Here's how the part is built. I have some questions about the finished solid (model axes, mm). A direction names the side the tool comes from. Coordinates: 2 decimals unless noted, no trailing zeros. Loops run counter-clockwise (first coordinate to the right, second up) from the corner with the lowest first, then second, coordinate; pieces in that order, holes last. Notation, with made-up numbers: (-31, 86.5) - (-26, 86.5) arc R35 ccw to (-26, 118.5) - close; hole circle Ø5 at (9, -16.5). An arc over 180 degrees is marked (long way). Use a Markdown table: item, result.
Autodesk Inventor part; units mm, degrees
ref_plane "YZ Plane" through (0, 0, 0) normal (1, 0, 0) x (0, 1, 0)
ref_plane "XZ Plane" through (0, 0, 0) normal (0, 1, 0) x (-1, 0, 0)
ref_plane "XY Plane" through (0, 0, 0) normal (0, 0, 1) x (1, 0, 0)
sketch "Sketch1" plane through (0, 0, 0) normal (0, 1, 0) x (-1, 0, 0)
  point P0 (0, 0)
sketch "Sketch2" plane through (0, 0, 0) normal (0, 1, 0) x (-1, 0, 0)
  line L0 (-76.2, 76.2) -> (76.2, 76.2)
  line L1 (76.2, 76.2) -> (76.2, -76.2)
  line L2 (76.2, -76.2) -> (-76.2, -76.2)
  line L3 (-76.2, -76.2) -> (-76.2, 76.2)
  line L4 (-76.2, 76.2) -> (76.2, -76.2) construction
  line L5 (76.2, 76.2) -> (-76.2, -76.2) construction
  point P0 (0, 0)
  dimension "d0" = 152.4
  dimension "d1" = 152.4
extrude "Extrusion1" add sketch "Sketch2" along normal blind 12.7
sketch "Sketch3" plane through (0, 12.7, 0) normal (0, 1, 0) x (1, 0, 0)
  line L0 (76.2, 76.2) -> (-76.2, 76.2)
  line L1 (76.2, -76.2) -> (76.2, 76.2)
  line L2 (-76.2, 76.2) -> (76.2, 76.2)
  line L3 (76.2, 76.2) -> (76.2, 63.5)
  line L4 (76.2, 63.5) -> (-76.2, 63.5)
  line L5 (-76.2, 63.5) -> (-76.2, 76.2)
  line L6 (-76.2, -76.2) -> (76.2, -76.2)
  line L7 (76.2, -76.2) -> (76.2, -63.5)
  line L8 (76.2, -63.5) -> (-76.2, -63.5)
  line L9 (-76.2, -63.5) -> (-76.2, -76.2)
  point P0 (0, 0)
  point P1 (76.2, -76.2)
  dimension "d4" = 12.7
  dimension "d5" = 12.7
  dimension "d15" = 152.4
extrude "Extrusion2" add sketch "Sketch3" along normal blind 127
fillet "Fillet1" radius 6.35 2 edges at (0, 0, 76.2) (0, 0, -76.2)
sketch "Sketch4" plane through (76.2, 12.7, -63.5) normal (1, 0, 0) x (0, 0, -1)
  circle A0 centre (-133.35, 120.65) radius 3.175
  circle A1 centre (-133.35, -6.35) radius 3.175
  circle A2 centre (-133.35, 57.15) radius 3.175
  circle A3 centre (6.35, 120.65) radius 3.175
  circle A4 centre (6.35, -6.35) radius 3.175
  circle A5 centre (6.35, 57.15) radius 3.175
  circle A6 centre (-63.5, -6.35) radius 3.175
  point P0 (-63.5, -12.7)
  dimension "d9" = 127
extrude "Extrusion3" cut sketch "Sketch4" against normal blind 12.7
sketch "Sketch5" plane through (-76.2, 12.7, 63.5) normal (-1, 0, 0) x (0, 0, 1)
  circle A0 centre (-133.35, 120.65) radius 3.175
  circle A1 centre (-133.35, 120.65) radius 3.175
  circle A2 centre (-133.35, 57.15) radius 3.175
  circle A3 centre (-133.35, 57.15) radius 3.175
  circle A4 centre (-133.35, -6.35) radius 3.175
  circle A5 centre (-133.35, -6.35) radius 3.175
  circle A6 centre (-63.5, -6.35) radius 3.175
  circle A7 centre (-63.5, -6.35) radius 3.175
  circle A8 centre (6.35, -6.35) radius 3.175
  circle A9 centre (6.35, -6.35) radius 3.175
  circle A10 centre (6.35, 57.15) radius 3.175
  circle A11 centre (6.35, 57.15) radius 3.175
  circle A12 centre (6.35, 120.65) radius 3.175
  circle A13 centre (6.35, 120.65) radius 3.175
  line L0 (6.35, -12.7) -> (-133.35, -12.7)
  point P0 (-63.5, -12.7)
  dimension "d20" = 69.85
sketch "Sketch6" plane through (0, 139.7, 0) normal (0, 1, 0) x (1, 0, 0)
  line L0 (76.2, 69.85) -> (-76.2, 69.85)
  circle A0 centre (0, 69.85) radius 3
  line L1 (-76.2, -69.85) -> (76.2, -69.85)
  circle A1 centre (0, -69.85) radius 3
  point P0 (0, 0)
  dimension "d16" = 6
  dimension "d17" = 6
extrude "Extrusion5" cut sketch "Sketch6" against normal blind 4
extrude "Extrusion6" cut sketch "Sketch5" against normal blind 12.7
properties part number "Fuselage_Body_Piece"
Q1. I want a section at A-A, the plane y = 133.35. Write out the boundary of the cut face in (x, z) (3 decimals).
Check values:
| item | result |
|---|---|
| outline | (-76.2, -76.2) - (76.2, -76.2) - (76.2, -73.025) - (63.5, -73.025) - (63.5, -66.675) - (76.2, -66.675) - (76.2, -63.5) - (-76.2, -63.5) - (-76.2, -66.675) - (-63.5, -66.675) - (-63.5, -73.025) - (-76.2, -73.025) - close; (-76.2, 63.5) - (76.2, 63.5) - (76.2, 66.675) - (63.5, 66.675) - (63.5, 73.025) - (76.2, 73.025) - (76.2, 76.2) - (-76.2, 76.2) - (-76.2, 73.025) - (-63.5, 73.025) - (-63.5, 66.675) - (-76.2, 66.675) - close |
Q2. I want a section at C-C, the plane z = 0. Write out the boundary of the cut face in (x, y) (3 decimals).
Check values:
| item | result |
|---|---|
| outline | (-76.2, 0) - (76.2, 0) - (76.2, 3.175) - (63.5, 3.175) - (63.5, 9.525) - (76.2, 9.525) - (76.2, 12.7) - (-76.2, 12.7) - (-76.2, 9.525) - (-63.5, 9.525) - (-63.5, 3.175) - (-76.2, 3.175) - close |
Q3. Which directions (+Z, -Z, +X, -X, +Y, -Y) give clear straight access to the entire face, cutting with the end or side of a thin tool? Please do faces 5 (the face through (63.5, 6, 70)), 6 (the face through (-69.94, 6.49, -73.02)), 7 (the face through (1, 75, 63.5)), 8 (the face through (0, 135.7, 70)).
Check values:
| item | result |
|---|---|
| face 5 | +X |
| face 6 | -X |
| face 7 | +X, -X, +Y |
| face 8 | +Y |
Q4. I want a section at B-B, the plane x = -9.5. Write out the boundary of the cut face in (y, z), then the cut area to 3 significant figures.
Check values:
| item | result |
|---|---|
| outline | (0, -69.85) arc R6.35 ccw to (6.35, -76.2) - (139.7, -76.2) - (139.7, -63.5) - (12.7, -63.5) - (12.7, 63.5) - (139.7, 63.5) - (139.7, 76.2) - (6.35, 76.2) arc R6.35 ccw to (0, 69.85) - close |
| area | 5,140 mm^2 |
Q5. Please list where these lines run through material, in increasing order: L1, parallel to Z at x = 73, y = 133; L2, parallel to Y at x = -67, z = -69.85 (3 decimals); L3, parallel to Z at x = 59.5, y = 43. Write a range as from..to.
Check values:
| item | result |
|---|---|
| L1 | -76.2..-73.01, -66.69..-63.5, 63.5..66.69, 73.01..76.2 |
| L2 | 0..3.175, 9.525..66.675, 73.025..130.175, 136.525..139.7 |
| L3 | -76.2..-63.5, 63.5..76.2 |
Q6. I want a section at D-D, the plane y = 47.5. Write out the boundary of the cut face in (x, z).
Check values:
| item | result |
|---|---|
| outline | (-76.2, -76.2) - (76.2, -76.2) - (76.2, -63.5) - (-76.2, -63.5) - close; (-76.2, 63.5) - (76.2, 63.5) - (76.2, 76.2) - (-76.2, 76.2) - close |
Q7. Will these pins go through, and if not, where does the flat tip stop? P1, Ø1.9, axis at y = 68.5, z = -70.5, coming from the -X side; P2, Ø5.5, axis at y = 133.35, z = 69.85, coming from the +X side.
Check values:
| item | result |
|---|---|
| P1 | x = -63.5 |
| P2 | x = 63.5 |
Q8. If we mould it in two halves opening along Y, with no side actions, what happens to faces 1 (the face through (69.94, 66.75, 70.54)), 2 (the face through (-0.391, 137.728, -72.824)), 3 (the face through (1, 12.7, 1)), 4 (the face through (69.939, 9.027, -1.707))? For each: pulls with the +Y half, pulls with the -Y half, needs draft (parallel to the pull), parting line crosses it, or undercut.
Check values:
| item | result |
|---|---|
| face 1 | undercut |
| face 2 | needs draft |
| face 3 | pulls with the +Y half |
| face 4 | undercut |
